```python
from build123d import *

# Parameters (mm, degrees)
SKETCH2_R           = 4
BOSS_EXTRUDE1_DEPTH = 115


with BuildPart() as part:
    # Sketch2 → Boss-Extrude1 (new body)
    with BuildSketch(Plane(origin=(0, 0, 0), x_dir=(1, 0, 0), z_dir=(0, 1, 0))):
        with Locations(Location((0, 0, 0), (0, 0, 270))):
            Circle(SKETCH2_R)
    extrude(amount=BOSS_EXTRUDE1_DEPTH)

    # Sketch5 → Ø3.0mm Dowel Hole1 (revolve, cut)
    with BuildSketch(Plane(origin=(0, 115, 0), x_dir=(0, 0, 1), z_dir=(1, 0, 0))):
        Polygon((0, 0), (0, 15.901290929), (1.5, 15), (1.5, 0.025), (1.525, 0), align=None)
    f_3_0mm_dowel_hole1 = revolve(axis=Axis((0, 121.35, 0), (0, -1, 0)), mode=Mode.SUBTRACT)

    # Mirror1: Ø3.0mm Dowel Hole1 across plane
    add(f_3_0mm_dowel_hole1.mirror(Plane.ZX.offset(57.5)), mode=Mode.SUBTRACT)


solid = part.part
```
Here's how the part is built. I have some questions about the finished solid (model axes, mm). A direction names the side the tool comes from. Coordinates: 2 decimals unless noted, no trailing zeros. Loops run counter-clockwise (first coordinate to the right, second up) from the corner with the lowest first, then second, coordinate; pieces in that order, holes last. Notation, with made-up numbers: (-6, -28) - (8, -28) arc R26 ccw to (8, 8) - close; hole circle Ø1 at (64, -9). An arc over 180 degrees is marked (long way). Answer as CSV lines item,"result".
Q1. For faces 1 (the face through (-0.07, 107.59, -1.5)), 2 (the face through (-0.07, 7.41, -1.5)), 3 (the face through (0, 115, 2)), which set-ups out of +Z, -Z, +X, -X, +Y, -Y let a thin tool reach every point of the face, with its end or its side?
Response:
face 1,"+Y"
face 2,"-Y"
face 3,"+Z, -Z, +X, -X, +Y"
Q2. If we section it at B-B, the plane x = -2.75: Write out the boundary of the cut face in (y, z).
Response:
outline,"(0, -2.9) - (115, -2.9) - (115, 2.9) - (0, 2.9) - close"
Q3. If I drill on L1, parallel to X at y = 105.75, z = 0; L2, parallel to Z at x = -3.5, y = 105.5; L3, parallel to Z at x = -1, y = 20.5, over which ranges is the centre line in solid material (lowest first)? Write a range as [from, to].
Response:
L1,"[-4, -1.5], [1.5, 4]"
L2,"[-1.94, 1.94]"
L3,"[-3.87, 3.87]"
Q4. We'd pull the mould along Z, two halves only. Please class faces 4 (the face through (0, 0, 2)), 5 (the face through (0.254, 99.255, -0.056)), 6 (the face through (-3.905, 56.695, -0.867)), 7 (the face through (0.231, 15.745, 0.12)): pulls with the +Z half, pulls with the -Z half, needs draft (parallel to the pull), parting line crosses it, or undercut.
Response:
face 4,"needs draft"
face 5,"undercut"
face 6,"parting line crosses it"
face 7,"undercut"
Q5. If we section it at A-A, the plane y = 95.5: Write out the boundary of the cut face in (x, z), and give its area (3 significant figures).
Response:
outline,"circle Ø8 at (0, 0)"
area,"50.3 mm2"
Q6. For pin 1 (2 mm diameter, centred on x = -2.5, y = 81.5, fed in from +Z); pin 2 (3 mm diameter, centred on x = 2.5, y = 18.5, fed in from -Z), each with a flat end and sliding along its axis, tell me the tip position at first contact or that it passes through.
Response:
pin 1,"z = 3.71"
pin 2,"z = -3.87"
Q7. If we section it at C-C, the plane z = 2.5: Write out the boundary of the cut face in (x, y).
Response:
outline,"(-3.12, 0) - (3.12, 0) - (3.12, 115) - (-3.12, 115) - close"
